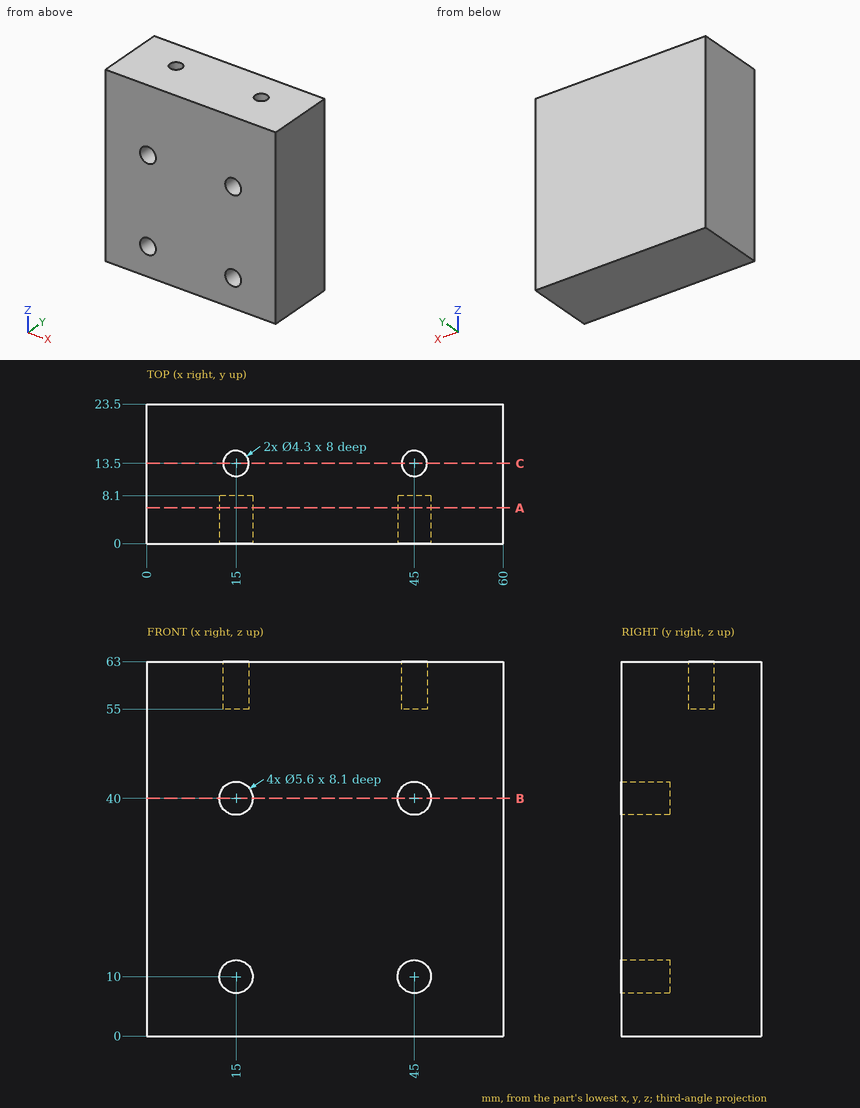
Geometry: see drawing. Coordinates: mm, zero at the bounding-box minimum. Coordinates: 2 decimals unless noted, no trailing zeros. Order: outer loops, then holes, each group sorted by start corner. A loop starts at its lowest first (then second) coordinate and runs counter-clockwise, first axis right, second up. Notation, with made-up numbers: (49, 37) - (71, 37) arc R20 ccw to (71, 70) - close; hole circle Ø1 at (88.25, -29). An arc over 180 degrees is marked (long way). Return JSON: item names as keys, results as strings.
Q1. Cut plane B-B (z = 40). Return loops of the section in (x, y).
The answers:
{"outline": "(0, 0) - (12.2, 0) - (12.2, 8.1) - (17.8, 8.1) - (17.8, 0) - (42.2, 0) - (42.2, 8.1) - (47.8, 8.1) - (47.8, 0) - (60, 0) - (60, 23.5) - (0, 23.5) - close"}
Q2. Ray query, probe 1 along X at (y, z) = (1.5, 10); probe 2 along Z at (x, y) = (42.5, 5.25); probe 3 along Y at (x, z) = (15, 60). Return the intervals inside material, ascending.
The answers:
{"probe 1": "x = 0 to 12.2, 17.8 to 42.2, 47.8 to 60", "probe 2": "z = 0 to 8.74, 11.26 to 38.74, 41.26 to 63", "probe 3": "y = 0 to 11.35, 15.65 to 23.5"}
Q3. Cut plane A-A (y = 6). Return loops of the section in (x, z).
The answers:
{"outline": "(0, 0) - (60, 0) - (60, 63) - (0, 63) - close; hole circle Ø5.6 at (15, 10); hole circle Ø5.6 at (15, 40); hole circle Ø5.6 at (45, 10); hole circle Ø5.6 at (45, 40)"}
Q4. Cut plane C-C (y = 13.5). Return loops of the section in (x, z).
The answers:
{"outline": "(0, 0) - (60, 0) - (60, 63) - (47.15, 63) - (47.15, 55) - (42.85, 55) - (42.85, 63) - (17.15, 63) - (17.15, 55) - (12.85, 55) - (12.85, 63) - (0, 63) - close"}
Q5. First-contact query: pin 1 (1.7 mm diameter, centred on x = 15, z = 10, fed in from -Y). Flat tip, straight axial feed; report the tip coordinate or a pass-through.
The answers:
{"pin 1": "stops at y = 8.1"}
